Can you work these out from the model? Positions are in its coordinate system, mm. Face numbers are marked on the shaded views. A direction names the side the tool comes from. Give positions to 0.01 mm unless a question says otherwise; leave off trailing zeros. Order: outer loops, then holes, each group sorted by start corner. A loop starts at its lowest first (then second) coordinate and runs counter-clockwise, first axis right, second up. Notation, with made-up numbers: M 4.5,-27.75 L 15.5,-27.75 A34 ccw 15.5,6.25 Z; hole C 10,32.25 d2. An arc over 180 degrees is marked long. Use one line per item in the form item = value. Start each with the question number.
1. I want a section at D-D, the plane x = 28. List the corners of the cut face in (y, z) for me.
2. For the marked faces 4, 5 and 6, which set-ups out of +Z, -Z, +X, -X, +Y, -Y let a thin tool reach every point of the face, with its end or its side?
3. I want a section at B-B, the plane y = 13. List the corners of the cut face in (x, z) for me.
4. We'd pull the mould along Y, two halves only. Please class the marked faces 1, 2 and 3: +Y half, -Y half, draft (parallel to the pull), parting line (faces both ways), or undercut.
5. I want a section at C-C, the plane x = 56. List the corners of the cut face in (y, z) for me.
6. Will these pins go through, and if not, where does the flat tip stop? P1, Ø2, axis at y = -55, z = -0.5, coming from the -X side; P2, Ø10.5, axis at x = 54.42, y = -46.21, coming from the +Z side; P3, Ø1, axis at y = -21.5, z = -2.5, coming from the -X side.
7. I want a section at A-A, the plane z = -0.75. List the corners of the cut face in (x, y) for me (3 decimals), and give its area (3 significant figures).
8. I need wall thicknesses on L1, parallel to X at y = -52, z = -1.75; L2, parallel to Y at x = 38, z = 2.25; L3, parallel to Y at x = 37, z = -2. Which ranges of each line are inside material? Lowest first, please.
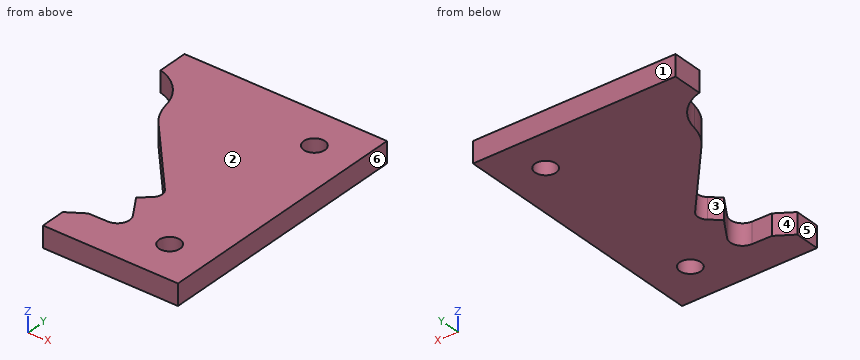
```python
from build123d import *

# Parameters (mm, degrees)
BOSS_EXTRUDE2_DEPTH        = 3.2893
FILLET4_R                  = 3.175
F_97_0_26_DIAMETER_HOLE1_D = 6.604


with BuildPart() as part:
    # Sketch1 → Boss-Extrude2 (new, symmetric)
    with BuildSketch(Plane.XY):
        with BuildLine():
            Line((40.245218881, -29.952840417), (34.814702315, -34.75119179))
            Line((34.814702315, -34.75119179), (36.859912069, -37.911424085))
            Line((36.859912069, -37.911424085), (39.325632445, -41.721424085))
            ThreePointArc((39.325632445, -41.721424085), (39.47389391, -45.61207473), (36.127033373, -47.601463693))
            Line((36.127033373, -47.601463693), (30.06004247, -47.717842457))
            Line((30.06004247, -47.717842457), (24.793517597, -51.126183057))
            Line((24.793517597, -51.126183057), (24.793517597, -58.914319794))
            Line((24.793517597, -58.914319794), (50.193517597, -58.914319794))
            Line((50.193517597, -58.914319794), (67.115922286, -58.914319794))
            Line((67.115922286, -58.914319794), (67.115922286, 23.635680206))
            Line((67.115922286, 23.635680206), (3.615922286, 23.635680206))
            Line((3.615922286, 23.635680206), (3.615922286, 14.236541628))
            ThreePointArc((3.615922286, 14.236541628), (10.763958516, 9.998143491), (14.46505327, 2.557690661))
            ThreePointArc((14.46505327, 2.557690661), (15.807885527, -1.447488843), (18.159107069, -4.956964385))
            Line((18.159107069, -4.956964385), (40.245218881, -29.952840417))
        make_face()
    extrude(amount=BOSS_EXTRUDE2_DEPTH, both=True)

    # Fillet4
    fillet4_edges = [part.edges().sort_by_distance(p)[0] for p in [
        (40.245218881, -29.952840417, 0),
    ]]
    fillet(fillet4_edges, radius=FILLET4_R)

    # #97 (0.26) Diameter Hole1 (through all)
    with Locations(Plane(origin=(54.415922286, 10.935680206, 3.2893), x_dir=(1, 0, 0), z_dir=(0, 0, 1))):
        with Locations((0, 0), (0, -57.15)):
            Hole(F_97_0_26_DIAMETER_HOLE1_D / 2)


solid = part.part
```
Check result:
q1.outline = M -58.91,-3.29 L -49.05,-3.29 L -49.05,3.29 L -58.91,3.29 Z; M -16.09,-3.29 L 23.64,-3.29 L 23.64,3.29 L -16.09,3.29 Z
q2.face_4 = +Z, -Z, -X
q2.face_5 = +Z, -Z, -X, -Y
q2.face_6 = +Z, -Z, +X, +Y, -Y
q3.outline = M 6.84,-3.29 L 51.84,-3.29 L 51.84,3.29 L 6.84,3.29 Z; M 56.99,-3.29 L 67.12,-3.29 L 67.12,3.29 L 56.99,3.29 Z
q4.face_1 = +Y half
q4.face_2 = draft
q4.face_3 = undercut
q5.outline = M -58.91,-3.29 L -49.11,-3.29 L -49.11,3.29 L -58.91,3.29 Z; M -43.32,-3.29 L 8.04,-3.29 L 8.04,3.29 L -43.32,3.29 Z; M 13.83,-3.29 L 23.64,-3.29 L 23.64,3.29 L 13.83,3.29 Z
q6.P1 = 24.79
q6.P2 = 3.29
q6.P3 = 32.33
q7.outline = M 3.616,14.237 A14.678 cw 14.465,2.558 A15.881 ccw 18.159,-4.957 L 38.143,-27.574 A3.175 cw 37.866,-32.055 L 34.815,-34.751 L 39.326,-41.721 A3.81 cw 36.127,-47.601 L 30.06,-47.718 L 24.794,-51.126 L 24.794,-58.914 L 67.116,-58.914 L 67.116,23.636 L 3.616,23.636 Z; hole C 54.416,-46.214 d6.604; hole C 54.416,10.936 d6.604
q7.area = 3,500 mm2
q8.L1 = 24.79 to 67.12
q8.L2 = -58.91 to -47.11, -39.67 to -31.93, -27.41 to 23.64
q8.L3 = -58.91 to -47.5, -38.13 to -32.82, -26.28 to 23.64
